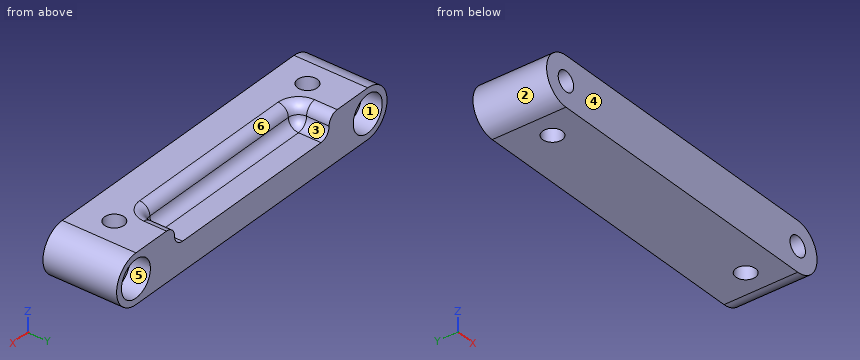
```python
from build123d import *

# Parameters (mm, degrees)
SKETCH1_R           = 2.4
BOSS_EXTRUDE1_DEPTH = 9
SKETCH2_R           = 4.5
CUT_EXTRUDE1_DEPTH  = 5
SKETCH3_W           = 48
SKETCH3_H           = 5
CUT_EXTRUDE2_DEPTH  = 8
FILLET1_R           = 2.5
SKETCH4_R           = 2.4
CUT_EXTRUDE3_DEPTH  = 45.598206242


with BuildPart() as part:
    # Sketch1 → Boss-Extrude1 (new, symmetric)
    with BuildSketch(Plane(origin=(0, 0, 0), x_dir=(1, 0, 0), z_dir=(0, 1, 0))):
        with BuildLine():
            Line((36, -6), (-36, -6))
            ThreePointArc((-36, -6), (-42, 0), (-36, 6))
            Line((-36, 6), (36, 6))
            ThreePointArc((36, 6), (42, 0), (36, -6))
        make_face()
        with Locations(Location((-36, 0, 0), (0, 0, 270))):
            Circle(SKETCH1_R, mode=Mode.SUBTRACT)
        with Locations(Location((36, 0, 0), (0, 0, 270))):
            Circle(SKETCH1_R, mode=Mode.SUBTRACT)
    extrude(amount=BOSS_EXTRUDE1_DEPTH, both=True)

    # Sketch2 → Cut-Extrude1 (cut)
    with BuildSketch(Plane(origin=(0, 9, 0), x_dir=(1, 0, 0), z_dir=(0, 1, 0))):
        with Locations(Location((-36, 0, 0), (0, 0, 270))):
            Circle(SKETCH2_R)
        with Locations(Location((36, 0, 0), (0, 0, 270))):
            Circle(SKETCH2_R)
    extrude(amount=-CUT_EXTRUDE1_DEPTH, mode=Mode.SUBTRACT)

    # Sketch3 → Cut-Extrude2 (cut)
    with BuildSketch(Plane(origin=(0, 9, 0), x_dir=(1, 0, 0), z_dir=(0, 1, 0))):
        with Locations((0, -3.5)):
            Rectangle(SKETCH3_W, SKETCH3_H)
    extrude(amount=-CUT_EXTRUDE2_DEPTH, mode=Mode.SUBTRACT)

    # Fillet1
    fillet1_edges = [part.edges().sort_by_distance(p)[0] for p in [
        (-24, 1, 3.5),
        (-24, 5, 6),
        (0, 1, 1),
        (-24, 5, 1),
        (24, 1, 3.5),
        (24, 5, 1),
        (0, 1, 6),
        (24, 5, 6),
    ]]
    fillet(fillet1_edges, radius=FILLET1_R - 0.0001)  # a hair under: the kernel refuses the full size

    # Sketch4 → Cut-Extrude3 (cut, through all)
    with BuildSketch(Plane.XY.offset(6)):
        with Locations((-30, -1)):
            Circle(SKETCH4_R)
        with Locations((30, -1)):
            Circle(SKETCH4_R)
    extrude(amount=-CUT_EXTRUDE3_DEPTH, mode=Mode.SUBTRACT)


solid = part.part
```
Geometry: final body of the model. Coordinates: model frame, mm. Face numbers are marked on the shaded views. A direction names the side the tool comes from. Round coordinates to 2 decimals unless told otherwise and drop trailing zeros. Order: outer loops, then holes, each group sorted by start corner. A loop starts at its lowest first (then second) coordinate and runs counter-clockwise, first axis right, second up. Notation, with made-up numbers: (28.5, 0.25) -> (42.5, 0.25) arc R14 cw to (42.5, 21.25) -> close; hole circle Ø9 at (-35.75, 22). An arc over 180 degrees is marked (long way). Use one line per item in the form item = value. Start each with the question number.
1. Pin query (flat end, axial travel): pin 1 Ø2.5 at (x, z) = (35.5, -0.5) entering from +Y; pin 2 Ø1.7 at (x, y) = (1.5, 6.5) entering from +Z; pin 3 Ø7 at (x, z) = (36, 0) entering from +Y; pin 4 Ø3 at (y, z) = (-3.5, 3) entering from -X. Return the tip coordinate at first contact, or that it passes through.
2. Draft query along Z for the marked faces 4, 5 and 6. Return one class per face: pulls with the +Z half, pulls with the -Z half, needs draft (parallel to the pull), parting line crosses it, or undercut.
3. Reachability of the marked faces 1, 2 and 3 from +Z, -Z, +X, -X, +Y, -Y: full face, straight path, thin tool, end or side. Return the list, or none.
4. Cut plane C-C (x = -30). Return the cut outline in (y, z), then the cut area to 3 significant figures.
5. Cut plane B-B (y = 6.25). Count the separate pieces of the cut face and the enclosed holes in it, then the cut area to 3 significant figures.
6. Line query: probe 1 along Y at (x, z) = (-30, -3.5); probe 2 along X at (y, z) = (1, -0.25); probe 3 along X at (y, z) = (-1.5, 3.5). Output: solid intervals per line, ascending.
7. Cut plane A-A (z = 0). Return the cut outline in (x, y), then the cut area to 3 significant figures.
Solution:
q1.pin_1 = through
q1.pin_2 = 1
q1.pin_3 = 4
q1.pin_4 = -41.81
q2.face_4 = needs draft
q2.face_5 = undercut
q2.face_6 = pulls with the +Z half
q3.face_1 = +Y
q3.face_2 = -X, +Y, -Y
q3.face_3 = +Z, +Y
q4.outline = (-9, -6) -> (-3.4, -6) -> (-3.4, 6) -> (-9, 6) -> close; (1.4, -6) -> (9, -6) -> (9, 6) -> (1.4, 6) -> close
q4.area = 158 mm^2
q5.separate_pieces = 1
q5.enclosed_holes = 2
q5.area = 610 mm^2
q6.probe_1 = -9 to -3.4, 1.4 to 9
q6.probe_2 = -41.99 to -38.39, -33.61 to -31.33, -28.67 to 28.67, 31.33 to 33.61, 38.39 to 41.99
q6.probe_3 = -40.87 to -32.35, -27.65 to 27.65, 32.35 to 40.87
q7.outline = (-42, -9) -> (-38.4, -9) -> (-38.4, 4) -> (-40.5, 4) -> (-40.5, 9) -> (-42, 9) -> close; (-33.6, -9) -> (33.6, -9) -> (33.6, 4) -> (31.5, 4) -> (31.5, 9) -> (-31.5, 9) -> (-31.5, 4) -> (-33.6, 4) -> close; (38.4, -9) -> (42, -9) -> (42, 9) -> (40.5, 9) -> (40.5, 4) -> (38.4, 4) -> close; hole circle Ø4.8 at (-30, -1); hole circle Ø4.8 at (30, -1)
q7.area = 1,260 mm^2
